Geometry check sheet. Reference: the model listing, model coordinates, mm. A direction names the side the tool comes from. Give positions to 0.01 mm unless a question says otherwise; leave off trailing zeros. Write each loop counter-clockwise with the first axis right and the second up, starting at its lowest first coordinate (ties: lowest second). Pieces come first, ordered by that corner, then holes. Notation, with made-up numbers: M 45.25,17 L 53.25,17 A20 cw 53.25,55 Z; hole C 31,-6.5 d10. An arc over 180 degrees is marked long. One line per item, written item: value. Start each with the question number.
1. Cross-section at C-C on z = -10.5. Record the cut outline in (x, y), then the cut area to 3 significant figures.
2. Tool access check on faces 4 (the face through (-157, 25, 51)), 5 (the face through (-157, 20.8, 58)), 6 (the face through (-162, 28, 20.65)). Record the directions out of +Z, -Z, +X, -X, +Y, -Y that give a thin tool (end or side, any length) a straight path to the whole face; none if there is none.
3. Release check for a two-part mould opening along Y. For faces 1 (the face through (-149, 18, 44)), 2 (the face through (-157, 7, 48)), 3 (the face through (-162, 15.8, 18)) record: pulls with the +Y half, pulls with the -Y half, needs draft (parallel to the pull), parting line crosses it, or undercut.
4. Scan lines: line 1 (X direction, y = 14.5, z = 4); line 2 (X direction, y = 32, z = 50); line 3 (Y direction, x = -60.5, z = 24). Record each from-to range of solid material in increasing order.
5. Gauge pin test, flat ends, axial feed: pin 1 (4 mm diameter, centred on x = -153, y = 9.5, fed in from -Z); pin 2 (4.5 mm diameter, centred on x = 27, z = 57, fed in from -Y); pin 3 (10 mm diameter, centred on x = -115, y = 6.5, fed in from -Z); pin 4 (1.6 mm diameter, centred on x = -161.5, y = 19, fed in from +Z). Record the tip position at first contact, or that the pin passes through.
6. Cross-section at B-B on y = 24. Record the cut outline in (x, z).
7. Cross-section at A-A on y = 11. Record the cut outline in (x, z).
8. Cross-section at D-D on x = 24.5. Record the cut outline in (y, z), then the cut area to 3 significant figures.
from build123d import *

# Parameters (mm, degrees)
SKETCH1_W           = 30
SKETCH1_H           = 30
BOSS_EXTRUDE1_DEPTH = 6
SKETCH2_W           = 30
SKETCH2_H           = 36
BOSS_EXTRUDE2_DEPTH = 6
SKETCH3_W           = 36
SKETCH3_H           = 36
BOSS_EXTRUDE3_DEPTH = 6
SKETCH4_W           = 36
SKETCH4_H           = 6
BOSS_EXTRUDE4_DEPTH = 165
SKETCH6_W           = 6
SKETCH6_H           = 30
BOSS_EXTRUDE6_DEPTH = 30
SKETCH9_W           = 6
SKETCH9_H           = 30
CUT_EXTRUDE2_DEPTH  = 20
SKETCH11_W          = 22
SKETCH11_H          = 5.2
SKETCH11_W_2        = 5.3
SKETCH11_H_2        = 15
CUT_EXTRUDE3_DEPTH  = 500
SKETCH13_W          = 16
SKETCH13_H          = 36
BOSS_EXTRUDE7_DEPTH = 30
SKETCH16_W          = 15
SKETCH16_H          = 5.3
CUT_EXTRUDE4_DEPTH  = 2090
SKETCH17_W          = 6
SKETCH17_H          = 36
BOSS_EXTRUDE8_DEPTH = 20


with BuildPart() as part:
    # Sketch1 → Boss-Extrude1 (new body)
    with BuildSketch(Plane(origin=(0, 0, 0), x_dir=(1, 0, 0), z_dir=(0, 1, 0))):
        with Locations((15, -15)):
            Rectangle(SKETCH1_W, SKETCH1_H)
    extrude(amount=BOSS_EXTRUDE1_DEPTH)

    # Sketch2 → Boss-Extrude2 (add)
    with BuildSketch(Plane(origin=(30, 0, 0), x_dir=(0, 0, -1), z_dir=(1, 0, 0))):
        with Locations((-15, 18)):
            Rectangle(SKETCH2_W, SKETCH2_H)
    extrude(amount=BOSS_EXTRUDE2_DEPTH)

    # Sketch3 → Boss-Extrude3 (add)
    with BuildSketch(Plane.XY.offset(30)):
        with Locations((18, 18)):
            Rectangle(SKETCH3_W, SKETCH3_H)
    extrude(amount=BOSS_EXTRUDE3_DEPTH)

    # Sketch4 → Boss-Extrude4 (add)
    with BuildSketch(Plane.ZY):
        with Locations((18, 3)):
            Rectangle(SKETCH4_W, SKETCH4_H)
    extrude(amount=BOSS_EXTRUDE4_DEPTH)

    # Sketch6 → Boss-Extrude6 (add)
    with BuildSketch(Plane(origin=(0, 6, 0), x_dir=(1, 0, 0), z_dir=(0, 1, 0))):
        Polygon((-165, -30), (-165, -36), (-149, -36), (-149, -30), (-159, -30), align=None)
        with Locations((-162, -15)):
            Rectangle(SKETCH6_W, SKETCH6_H)
    extrude(amount=BOSS_EXTRUDE6_DEPTH)

    # Sketch9 → Cut-Extrude2 (cut)
    with BuildSketch(Plane.ZY):
        with Locations((33, 21)):
            Rectangle(SKETCH9_W, SKETCH9_H)
    extrude(amount=-CUT_EXTRUDE2_DEPTH, mode=Mode.SUBTRACT)

    # Sketch11 → Cut-Extrude3 (cut)
    with BuildSketch(Plane(origin=(36, 0, 0), x_dir=(0, 0, -1), z_dir=(1, 0, 0))):
        with Locations((-18, 18.4)):
            Rectangle(SKETCH11_W, SKETCH11_H)
        with Locations((-18, 28.5)):
            Rectangle(SKETCH11_W_2, SKETCH11_H_2)
    extrude(amount=-CUT_EXTRUDE3_DEPTH, mode=Mode.SUBTRACT)

    # Sketch13 → Boss-Extrude7 (add)
    with BuildSketch(Plane.XY.offset(36)):
        with Locations((-157, 18)):
            Rectangle(SKETCH13_W, SKETCH13_H)
        with Locations((28, 18)):
            Rectangle(SKETCH13_W, SKETCH13_H)
    extrude(amount=BOSS_EXTRUDE7_DEPTH)

    # Sketch16 → Cut-Extrude4 (cut)
    with BuildSketch(Plane.ZY.offset(165)):
        Polygon((51, 15.5), (51, 20.8), (51, 29), (45.8, 29), (45.8, 7), (51, 7), align=None)
        with Locations((58.5, 18.15)):
            Rectangle(SKETCH16_W, SKETCH16_H)
    extrude(amount=-CUT_EXTRUDE4_DEPTH, mode=Mode.SUBTRACT)

    # Sketch17 → Boss-Extrude8 (add)
    with BuildSketch(Plane(origin=(0, 0, 0), x_dir=(-1, 0, 0), z_dir=(0, 0, -1))):
        Polygon((159, 6), (159, 0), (165, 0), (165, 36), (159, 36), align=None)
        with Locations((-33, 18)):
            Rectangle(SKETCH17_W, SKETCH17_H)
    extrude(amount=BOSS_EXTRUDE8_DEPTH)


solid = part.part
Report:
1. outline: M -165,0 L -159,0 L -159,36 L -165,36 Z; M 30,0 L 36,0 L 36,36 L 30,36 Z
1. area: 432 mm^2
2. face 4: +X, -X
2. face 5: +Z, +X, -X
2. face 6: +X, -X, +Y
3. face 1: needs draft
3. face 2: undercut
3. face 3: undercut
4. line 1: x = -165 to -159, 30 to 36
4. line 2: x = -165 to -149, 20 to 36
4. line 3: y = 0 to 6
5. pin 1: stops at z = 30
5. pin 2: stops at y = 0
5. pin 3: stops at z = 0
5. pin 4: stops at z = 45.8
6. outline: M -165,-20 L -159,-20 L -159,15.35 L -165,15.35 Z; M -165,20.65 L -159,20.65 L -159,30 L -149,30 L -149,45.8 L -165,45.8 Z; M -165,51 L -149,51 L -149,66 L -165,66 Z; M 20,30 L 30,30 L 30,20.65 L 36,20.65 L 36,45.8 L 20,45.8 Z; M 20,51 L 36,51 L 36,66 L 20,66 Z; M 30,-20 L 36,-20 L 36,15.35 L 30,15.35 Z
7. outline: M -165,-20 L -159,-20 L -159,30 L -149,30 L -149,45.8 L -165,45.8 Z; M -165,51 L -149,51 L -149,66 L -165,66 Z; M 20,30 L 30,30 L 30,-20 L 36,-20 L 36,45.8 L 20,45.8 Z; M 20,51 L 36,51 L 36,66 L 20,66 Z
8. outline: M 0,0 L 6,0 L 6,30 L 36,30 L 36,66 L 20.8,66 L 20.8,51 L 29,51 L 29,45.8 L 7,45.8 L 7,51 L 15.5,51 L 15.5,66 L 0,66 Z
8. area: 1,280 mm^2
